from build123d import *

# Parameters (mm, degrees)
F1_DEPTH = 25.4
F3_DEPTH = 30
F4_DEPTH = 30
F7_DEPTH = 25
F9_DEPTH = 40
F11_SIZE = 5
F12_SIZE = 3
F13_SIZE = 1.5


# Not quite as in the source:
# - a feature of the source that left no trace in its solid (it failed there, or was rolled back) is left out


with BuildPart() as f1:
    # F0 (on Front) → F1 (new body)
    with BuildSketch(Plane.XZ):
        Polygon((10.4166865349, 52.9566034675), (-31.557098031, 52.9566034675), (-31.557098031, 0), (-18.2580947876, -28.9524644613), (-18.2580947876, -36.2323522568), (-10.9038203955, -36.2323522568), (-10.9038203955, -45.4944968224), (0, -54.6278357506), (10.4166865349, -54.6278357506), align=None)
    extrude(amount=F1_DEPTH)


with BuildPart() as f3:
    # F2 (on Front) → F3 (new body, symmetric)
    with BuildSketch(Plane.XZ):
        with BuildLine():
            Line((-19.7998397052, 47.9566034675), (-26.557098031, 47.9566034675))
            Line((-26.557098031, 47.9566034675), (-26.557098031, 30.8428518474))
            Line((-26.557098031, 30.8428518474), (-21.0963413119, 30.8428518474))
            Line((-21.0963413119, 30.8428518474), (-21.0963413119, 12.7346292138))
            Line((-21.0963413119, 12.7346292138), (-26.557098031, 12.7346292138))
            Line((-26.557098031, 12.7346292138), (-26.557098031, 1.0934300149))
            Line((-26.557098031, 1.0934300149), (-22.3559527725, -8.0526320297))
            Line((-22.3559527725, -8.0526320297), (-17.2149640966, -6.7084824335))
            Line((-17.2149640966, -6.7084824335), (-13.8887305603, 1.4067513807))
            ThreePointArc((-13.8887305603, 1.4067513807), (-14.1854089296, 10.908286), (-5.9038203955, 6.2411166728))
            ThreePointArc((-5.9038203955, 6.2411166728), (-5.9071677422, 6.0500291804), (-5.9172056749, 5.8591761626))
            Line((-5.9172056749, 5.8591761626), (2.6482306421, 5.8591761626))
            Line((2.6482306421, 5.8591761626), (2.6482306421, 37.4990403652))
            Line((2.6482306421, 37.4990403652), (5.4166865349, 37.4990403652))
            Line((5.4166865349, 37.4990403652), (5.4166865349, 47.9566034675))
            Line((5.4166865349, 47.9566034675), (0, 47.9566034675))
            Line((0, 47.9566034675), (0, 41.127063334))
            Line((0, 41.127063334), (-19.7998397052, 41.127063334))
            Line((-19.7998397052, 41.127063334), (-19.7998397052, 47.9566034675))
        make_face()
    extrude(amount=F3_DEPTH, both=True)


with BuildPart() as f4:
    # F2 (on Front) → F4 (new body, symmetric)
    with BuildSketch(Plane.XZ):
        with BuildLine():
            Line((-16.1110319639, -7.9702737021), (-21.7201422185, -9.4368171549))
            Line((-21.7201422185, -9.4368171549), (-13.2580947876, -27.8590344464))
            Line((-13.2580947876, -27.8590344464), (-13.2580947876, -31.2323522568))
            Line((-13.2580947876, -31.2323522568), (-5.9038203955, -31.2323522568))
            Line((-5.9038203955, -31.2323522568), (-5.9038203955, -43.1603266307))
            Line((-5.9038203955, -43.1603266307), (1.8174038362, -49.6278357506))
            Line((1.8174038362, -49.6278357506), (5.4166865349, -49.6278357506))
            Line((5.4166865349, -49.6278357506), (5.4166865349, -39.5213142037))
            Line((5.4166865349, -39.5213142037), (2.6482306421, -39.5213142037))
            Line((2.6482306421, -39.5213142037), (2.6482306421, 4.3591761626))
            Line((2.6482306421, 4.3591761626), (-6.238670659, 4.3591761626))
            ThreePointArc((-6.238670659, 4.3591761626), (-8.7135994884, 1.4698551421), (-12.4751443179, 0.900443897))
            Line((-12.4751443179, 0.900443897), (-16.1110319639, -7.9702737021))
        make_face()
    extrude(amount=F4_DEPTH, both=True)


with BuildPart() as f1_1:
    add(f1.part)

    # F5: cut F3
    add(f3.part, mode=Mode.SUBTRACT)

    # F6: cut F4
    add(f4.part, mode=Mode.SUBTRACT)

    # F7 (add): a face of the model
    f7_faces = [f1_1.faces().sort_by_distance(p)[0] for p in [
        (-7.5880887423, 0, 6.6814576026),
    ]]
    extrude(f7_faces, amount=F7_DEPTH)


with BuildPart() as f9:
    # F8 (on Right) → F9 (new body, symmetric)
    with BuildSketch(Plane.YZ):
        Polygon((-5.4386107326, 32.0926371886), (-5.4386107326, 63.2104203105), (-7.4386107326, 63.2104203105), (-7.4386107326, 32.5547352223), (-14.0266608968, 19.0589928517), (-14.0266608968, -19.9610399589), (-3.9184388004, -59.6407970668), (-1.9803369667, -59.1470751993), (-12.0266608968, -19.7102989226), (-12.0266608968, 18.596894818), align=None)
    extrude(amount=F9_DEPTH, both=True)


with BuildPart() as f1_2:
    add(f1_1.part)

    # F10: intersect F9
    add(f9.part, mode=Mode.INTERSECT)

    # F11
    f11_edges = [f1_2.edges().sort_by_distance(p)[0] for p in [
        (-26.557098, -6.438611, 47.956603),
        (10.416687, -6.438611, 52.956603),
        (-31.557098, -6.438611, 52.956603),
        (0, -6.438611, 41.127063),
        (-19.79984, -6.438611, 41.127063),
        (-21.096341, -13.026661, 12.734629),
    ]]
    chamfer(f11_edges, length=F11_SIZE)

    # F12
    f12_edges = [f1_2.edges().sort_by_distance(p)[0] for p in [
        (5.416687, -6.438611, 47.956603),
        (-21.096341, -7.161491, 30.842852),
        (5.416687, -5.437254, -49.627836),
        (-5.90382, -10.123412, -31.232352),
        (-13.258095, -10.123412, -31.232352),
    ]]
    chamfer(f12_edges, length=F12_SIZE)

    # F13
    f13_edges = [f1_2.edges().sort_by_distance(p)[0] for p in [
        (2.648231, -6.438611, 37.49904),
    ]]
    chamfer(f13_edges, length=F13_SIZE)


solid = f1_2.part
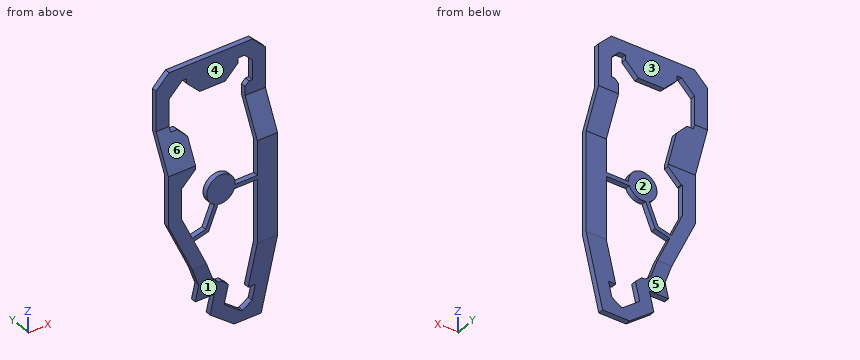
Geometry: final body of the model. Coordinates: model frame, mm. Face numbers are marked on the shaded views. A direction names the side the tool comes from. Give positions to 0.01 mm unless a question says otherwise; leave off trailing zeros. Loops run counter-clockwise (first coordinate to the right, second up) from the corner with the lowest first, then second, coordinate; pieces in that order, holes last. Notation, with made-up numbers: M -18,-19.75 L -14,-19.75 A10 cw -14,-8.75 Z; hole C 79.5,-26.75 d11. An arc over 180 degrees is marked long. Put each result on its own line as item: value. Start each with the question number.
1) Cut plane B-B (z = -2). Output: boundary loops of the cut face in (x, y).
2) Access query for the marked faces 1, 2 and 3. Directions: +Z, -Z, +X, -X, +Y, -Y. A direction counts if a zero-diameter tool reaches every point of the face in a straight line with its end or side. Return the directions, or none.
3) Ray query, line 1 along Y through (x, z) = (4.5, -12); line 2 along Y through (x, z) = (-29, 45); line 3 along Z through (x, y) = (-28, -8). Return the intervals inside material, ascending.
4) Cut plane A-A (z = 34). Output: boundary loops of the cut face in (x, y).
5) Contact query for flat-ended pins moving along their axis: pin 1 (1 mm diameter, centred on x = -1, y = -13, fed in from -Z); pin 2 (1.2 mm diameter, centred on y = -7, z = -42.5, fed in from -X); pin 3 (0.6 mm diameter, centred on x = 3.5, y = -8.5, fed in from -Z). Output: stop coordinate, or through.
6) Pull-direction query (Z, two-part tool) for the marked faces 4, 5 and 6; classes: pulls with the +Z half, pulls with the -Z half, needs draft (parallel to the pull), parting line crosses it, or undercut.
Verdict:
1. outline: M -30.64,-14.03 L -25.14,-14.03 L -25.14,-12.03 L -30.64,-12.03 Z; M -15.29,-14.03 L -13.66,-14.03 L -13.66,-12.03 L -15.29,-12.03 Z; M 2.65,-14.03 L 10.42,-14.03 L 10.42,-12.03 L 2.65,-12.03 Z
2. face 1: -Z, +X, -X, -Y
2. face 2: +X, -X, +Y
2. face 3: +Z, +X, -X, +Y
3. line 1: -14.03 to -12.03
3. line 2: -7.44 to -5.44
3. line 3: 26.85 to 31.4
4. outline: M -31.56,-7.44 L -26.56,-7.44 L -26.56,-5.44 L -31.56,-5.44 Z; M 2.65,-7.44 L 10.42,-7.44 L 10.42,-5.44 L 2.65,-5.44 Z
5. pin 1: z = 4.36
5. pin 2: x = -10.9
5. pin 3: z = -39.52
6. face 4: needs draft
6. face 5: undercut
6. face 6: pulls with the +Z half
